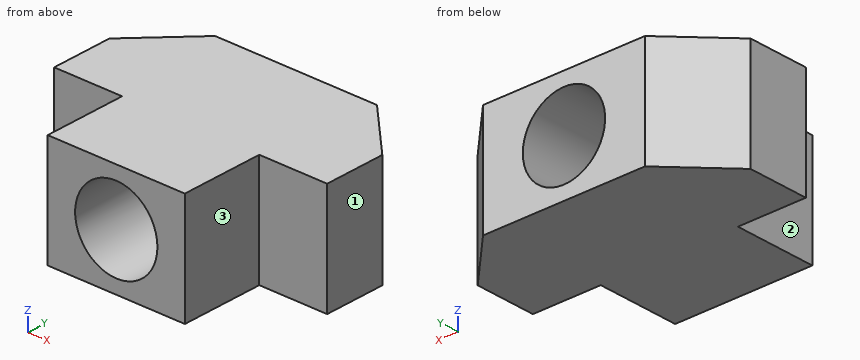
from build123d import *

# Parameters (mm, degrees)
EXTRUDE1_DEPTH     = 4
CUT_EXTRUDE1_REACH = 20.035
SKETCH2_R          = 3


with BuildPart() as part:
    # Sketch1 → Extrude1 (new, symmetric)
    with BuildSketch(Plane.XY):
        Polygon((-5, 0), (5, 0), (5, 6), (9.95, 6), (9.95, 10.45), (5.9, 14.5), (-5.9, 14.5), (-9.95, 10.45), (-9.95, 6), (-5, 6), align=None)
    extrude(amount=EXTRUDE1_DEPTH, both=True)

    # Sketch2 → Cut-Extrude1 (cut, up to next)
    with BuildSketch(Plane(origin=(0, 0, 0), x_dir=(1, 0, 0), z_dir=(0, 1, 0)), mode=Mode.PRIVATE) as cut_extrude1_sk1:
        Circle(SKETCH2_R)
    cut_extrude1_tool1 = extrude(cut_extrude1_sk1.sketch, amount=CUT_EXTRUDE1_REACH, mode=Mode.PRIVATE) & part.part
    add(cut_extrude1_tool1.solids().sort_by_distance((0, 0, 0))[0], mode=Mode.SUBTRACT)


solid = part.part
Could you check a few things on this model? Use its own coordinates, in mm. Face numbers are marked on the shaded views. A direction names the side the tool comes from. Coordinates: 2 decimals unless noted, no trailing zeros. Write each loop counter-clockwise with the first axis right and the second up, starting at its lowest first coordinate (ties: lowest second). Pieces come first, ordered by that corner, then holes. Notation, with made-up numbers: (67, 45.5) - (90, 45.5) arc R25 cw to (90, 72.5) - close; hole circle Ø5 at (-14.5, 33.5). An arc over 180 degrees is marked (long way). Write item = value, one per line.
1) Will these pins go through, and if not, where does the flat tip stop? pin 1 Ø2.5 at (x, z) = (-7.5, -1) entering from -Y; pin 2 Ø1.5 at (x, y) = (6.5, 3) entering from -Z; pin 3 Ø3 at (y, z) = (4, -1.5) entering from +X.
Result set:
pin_1 = 6
pin_2 = through
pin_3 = 5
2) Please list where these lines run through material, in increasing order: line 1 (Z direction, x = 0, y = 6.75); line 2 (X direction, y = 4.75, z = 0); line 3 (X direction, y = 10, z = 0). Write a range as [from, to].
Result set:
line_1 = [-4, -3], [3, 4]
line_2 = [-5, -3], [3, 5]
line_3 = [-9.95, -3], [3, 9.95]
3) Suppose I cut it at A-A on x = 0. Please give me the cut outline in (y, z), plus the area to 3 significant figures.
Result set:
outline = (0, -4) - (14.5, -4) - (14.5, -3) - (0, -3) - close; (0, 3) - (14.5, 3) - (14.5, 4) - (0, 4) - close
area = 29.0 mm2
4) Suppose I cut it at C-C on y = 5.25. Please give me the cut outline in (x, z).
Result set:
outline = (-5, -4) - (5, -4) - (5, 4) - (-5, 4) - close; hole circle Ø6 at (0, 0)
5) Suppose I cut it at D-D on z = -2.25. Please give me the cut outline in (x, y).
Result set:
outline = (-9.95, 6) - (-5, 6) - (-5, 0) - (-1.98, 0) - (-1.98, 14.5) - (-5.9, 14.5) - (-9.95, 10.45) - close; (1.98, 0) - (5, 0) - (5, 6) - (9.95, 6) - (9.95, 10.45) - (5.9, 14.5) - (1.98, 14.5) - close
6) Suppose I cut it at B-B on z = 0. Please give me the cut outline in (x, y).
Result set:
outline = (-9.95, 6) - (-5, 6) - (-5, 0) - (-3, 0) - (-3, 14.5) - (-5.9, 14.5) - (-9.95, 10.45) - close; (3, 0) - (5, 0) - (5, 6) - (9.95, 6) - (9.95, 10.45) - (5.9, 14.5) - (3, 14.5) - close
7) For the marked faces 1, 2 and 3, which set-ups out of +Z, -Z, +X, -X, +Y, -Y let a thin tool reach every point of the face, with its end or its side?
Result set:
face_1 = +Z, -Z, +X, +Y, -Y
face_2 = +Z, -Z, -X, -Y
face_3 = +Z, -Z, +X, -Y
